Autodesk Inventor part; units mm, degrees
ref_plane "YZ Plane" through (0, 0, 0) normal (1, 0, 0) x (0, 1, 0)
ref_plane "XZ Plane" through (0, 0, 0) normal (0, 1, 0) x (-1, 0, 0)
ref_plane "XY Plane" through (0, 0, 0) normal (0, 0, 1) x (1, 0, 0)
sketch "Sketch2" plane through (0, 0, 0) normal (0, 0, 1) x (1, 0, 0)
  line L0 (1.043, 0.3192) -> (1.043, -4.0683)
  arc A0 (1.043, 0.3192) -> (-5.457, 0.3192) centre (-2.207, 3.4317) ccw
  circle A1 centre (-2.207, -4.0683) radius 3.25
  circle A2 centre (-2.207, 3.4317) radius 3.25
  line L1 (-2.207, 14.5026) -> (-2.207, -15.0875) construction
  line L2 (-5.457, 0.3192) -> (-5.457, -4.0683)
  point P0 (-2.7063, -6.309)
  dimension "d6" = 6.5
  dimension "d8" = 9
  dimension "d9" = 7.5
extrude "Extrusion1" add sketch "Sketch2" along normal blind 5 contours A1
extrude "Extrusion2" add sketch "Sketch2" against normal blind 10 contours L0 A1 L2 A0 | A1 | A2
sketch "Sketch3" plane through (0, 0, -10) normal (0, 0, -1) x (-1, 0, 0)
  circle A0 centre (2.207, 3.4317) radius 3.25
  arc A1 (5.457, 0.3192) -> (-1.043, 0.3192) centre (2.207, 3.4317) ccw
  point P0 (0, 0)
extrude "Extrusion3" add sketch "Sketch3" along normal blind 5
equation "\"d6\" = R"
equation "\"d8\" = R1"
equation "\"d0\" = thickness"
equation "\"d2\" = 2 * thickness"
equation "\"d4\" = thickness"
equation "\"R\" = 6.5"
equation "\"thickness\" = 5"
equation "\"width\" = 6.5"
equation "\"R1\" = 9"
Geometry check sheet. Reference: the model listing, model coordinates, mm. A direction names the side the tool comes from. Coordinates: 2 decimals unless noted, no trailing zeros. Order: outer loops, then holes, each group sorted by start corner. A loop starts at its lowest first (then second) coordinate and runs counter-clockwise, first axis right, second up.
Q1. Tool access check on faces 5 (the face through (-2, -1, -10)), 6 (the face through (-2, -4, 5)), 7 (the face through (-2.63, -7.29, -0.94)). Record the directions out of +Z, -Z, +X, -X, +Y, -Y that give a thin tool (end or side, any length) a straight path to the whole face; none if there is none.
Reply:
face 5: -Z
face 6: +Z, +X, -X, +Y, -Y
face 7: +Z
Q2. Draft check along X on faces 1 (the face through (1.043, -2, -5)), 2 (the face through (0.188, 1.235, -12.465)), 3 (the face through (-5.457, -2, -5)), 4 (the face through (-2, 3, -15)). Enter one of: released by +X, released by -X, zero draft, split by the parting line, or undercut.
Reply:
face 1: released by +X
face 2: split by the parting line
face 3: released by -X
face 4: zero draft
Q3. Sectioned sample at D-D on y = 5.25. Record the cut outline in (x, z).
Reply:
outline: (-6.32, -10) - (-4.9, -10) - (-4.9, -15) - (0.49, -15) - (0.49, -10) - (1.91, -10) - (1.91, 0) - (-6.32, 0) - close
Q4. Sectioned sample at C-C on x = -4. Record the cut outline in (y, z), and give its area (3 significant figures).
Reply:
outline: (-6.78, -10) - (0.72, -10) - (0.72, -15) - (6.14, -15) - (6.14, -10) - (7.56, -10) - (7.56, 0) - (-1.36, 0) - (-1.36, 5) - (-6.78, 5) - close
area: 198 mm2
Q5. Sectioned sample at A-A on x = -2. Record the cut outline in (y, z).
Reply:
outline: (-7.31, -10) - (0.19, -10) - (0.19, -15) - (6.68, -15) - (6.68, -10) - (7.93, -10) - (7.93, 0) - (-0.82, 0) - (-0.82, 5) - (-7.31, 5) - close
Q6. Sectioned sample at B-B on y = -3.5. Record the cut outline in (x, z), and give its area (3 significant figures).
Reply:
outline: (-5.46, -10) - (1.04, -10) - (1.04, 0) - (0.99, 0) - (0.99, 5) - (-5.41, 5) - (-5.41, 0) - (-5.46, 0) - close
area: 97.0 mm2
Q7. Thickness scan on probe 1 along Z at (x, y) = (-1, -4.5); probe 2 along Z at (x, y) = (-5.5, 2.25); probe 3 along X at (y, z) = (-4.25, -9.25). Record the ranges inside material, lowest first.
Reply:
probe 1: z = -10 to 5
probe 2: z = -10 to 0
probe 3: x = -5.45 to 1.04
Q8. Depth check by flat-ended pin: pin 1 Ø1.3 at (y, z) = (-1.5, -6) entering from +X; pin 2 Ø2 at (y, z) = (-2.5, -3) entering from -X; pin 3 Ø1 at (x, y) = (-3.5, -0.5) entering from +Z. Enter the tip coordinate at first touch or a pass-through.
Reply:
pin 1: stops at x = 1.04
pin 2: stops at x = -5.46
pin 3: stops at z = 0
